Input: part model. Units: mm. Frame: model coordinates. Face numbers are marked on the shaded views. A direction names the side the tool comes from. Coordinates: 2 decimals unless noted, no trailing zeros. Write each loop counter-clockwise with the first axis right and the second up, starting at its lowest first coordinate (ties: lowest second). Pieces come first, ordered by that corner, then holes. Notation, with made-up numbers: (41.25, 74) - (100.25, 74) arc R11 cw to (100.25, 82) - close; hole circle Ø9 at (12.25, 77.25). An arc over 180 degrees is marked (long way). Use CSV: the item, a comma, the result in double quotes.
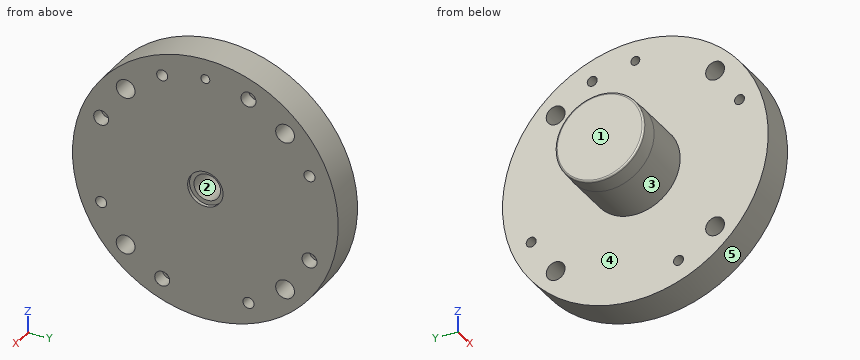
```python
from build123d import *

# Parameters (mm, degrees)
F2_R             = 6.7437
F3_DEPTH         = 25.4
F3_COPIES_COUNT  = 4
F8_COPIES_COUNT  = 4
F11_COPIES_COUNT = 4
F12_R            = 3.175
F13_DEPTH        = 25.4


# Not quite as in the source:
# - a pattern or mirror of a feature is missing from the dataset's text; its kind, count and spacing are read off the source's solid


with BuildPart() as f1:
    # F0 (on Front) → F1 (revolve)
    with BuildSketch(Plane.XZ):
        with BuildLine():
            Line((-46.99, 30.4610814834), (-46.99, 0))
            Line((-46.99, 0), (25.4, 0))
            Line((25.4, 0), (25.4, 95.25))
            Line((25.4, 95.25), (0, 95.25))
            Line((0, 95.25), (0, 32.131))
            Line((0, 32.131), (-34.29, 32.131))
            Line((-34.29, 32.131), (-45.7643223608, 31.7303078338))
            ThreePointArc((-45.7643223608, 31.7303078338), (-46.6335615464, 31.3432976139), (-46.99, 30.4610814834))
        make_face()
    revolve(axis=Axis((-33.2340214019, 0, 0), (-1, 0, 0)))

    # F2 (on Right) → F3 (cut, through all)
    with BuildSketch(Plane.YZ):
        with Locations((57.15, 57.15)):
            Circle(F2_R)
    f3 = extrude(amount=F3_DEPTH, mode=Mode.SUBTRACT)

    # F3_copies: F3 ×4 about axis
    f3_copies_axis = Axis((0, 0, 0), (1, 0, 0))
    for i in range(1, F3_COPIES_COUNT):
        add(f3.rotate(f3_copies_axis, i * 360 / F3_COPIES_COUNT), mode=Mode.SUBTRACT)

    # F4 (on Front) → F5 (revolve, cut)
    with BuildSketch(Plane.XZ):
        Polygon((-38.0918026038, 9.525), (-43.815, 0), (25.4, 0), (25.4, 12.7), (22.86, 12.7), (22.86, 9.525), align=None)
    revolve(axis=Axis((25.4, 0, 0), (1, 0, 0)), mode=Mode.SUBTRACT)

    # F7 (on line) → F8 (revolve, cut)
    with BuildSketch(Plane(origin=(0, 0, 0), x_dir=(-1, 0, 0), z_dir=(0, 0.9238795325, -0.3826834324))):
        Polygon((-25.4, 80.8228), (0, 80.8228), (0, 84.3915), (-15.494, 84.3915), (-15.494, 86.1822), (-25.4, 86.1822), align=None)
    f8 = revolve(axis=Axis((19.0941668783, 30.9295465174, 74.6705306803), (-1, 0, 0)), mode=Mode.SUBTRACT)

    # F8_copies: F8 ×4 about axis
    f8_copies_axis = Axis((0, 0, 0), (1, 0, 0))
    for i in range(1, F8_COPIES_COUNT):
        add(f8.rotate(f8_copies_axis, i * 360 / F8_COPIES_COUNT), mode=Mode.SUBTRACT)

    # F10 (on line) → F11 (revolve, cut)
    with BuildSketch(Plane(origin=(0, 0, 0), x_dir=(-1, 0, 0), z_dir=(0, 0.9238795325, 0.3826834324))):
        Polygon((-25.4, 84.79155), (-25.4, 80.8228), (-2.9182675346, 80.8228), (-4.826, 83.9978), (-7.9248, 83.9978), (-7.9248, 84.79155), align=None)
    f11 = revolve(axis=Axis((19.9955312124, -30.9295465174, 74.6705306803), (-1, 0, 0)), mode=Mode.SUBTRACT)

    # F11_copies: F11 ×4 about axis
    f11_copies_axis = Axis((0, 0, 0), (1, 0, 0))
    for i in range(1, F11_COPIES_COUNT):
        add(f11.rotate(f11_copies_axis, i * 360 / F11_COPIES_COUNT), mode=Mode.SUBTRACT)

    # F12 (on Right) → F13 (cut, through all)
    with BuildSketch(Plane.YZ):
        with Locations((0, 80.8228)):
            Circle(F12_R)
    extrude(amount=F13_DEPTH, mode=Mode.SUBTRACT)


solid = f1.part
```
(1) Reachability of the marked faces 4 and 5 from +Z, -Z, +X, -X, +Y, -Y: full face, straight path, thin tool, end or side. Return the list, or none.
Check values:
face 4,"-X"
face 5,"+X, -X"
(2) Cut plane A-A on z = 57.15. Return loops of the section in (x, y), and give its area (3 significant figures).
Check values:
outline,"(0, -76.2) - (25.4, -76.2) - (25.4, -63.89) - (0, -63.89) - close; (0, -50.41) - (25.4, -50.41) - (25.4, 50.41) - (0, 50.41) - close; (0, 63.89) - (25.4, 63.89) - (25.4, 76.2) - (0, 76.2) - close"
area,"3,190 mm^2"
(3) Cut plane C-C on x = 19. State how many separate pieces and enclosed holes the cut face has, and give its area (3 significant figures).
Check values:
separate pieces,"1"
enclosed holes,"14"
area,"27,100 mm^2"
(4) Ray query, probe 1 along Y at (x, z) = (9, 56.5); probe 2 along Z at (x, y) = (-17.5, 29.5); probe 3 along X at (y, z) = (49.5, -64). Return the intervals inside material, ascending. Write a range as from..to.
Check values:
probe 1,"-76.68..-63.86, -50.44..50.44, 63.86..76.68"
probe 2,"-12.73..12.73"
probe 3,"0..25.4"
(5) Pin query (flat end, axial travel): pin 1 Ø4 at (x, y) = (-38.5, 7) entering from +Z; pin 2 Ø2 at (x, y) = (-36, 14.5) entering from +Z; pin 3 Ø8 at (y, z) = (6, -3) entering from +X. Return the tip coordinate at first contact, or that it passes through.
Check values:
pin 1,"z = 31.6"
pin 2,"z = 29.09"
pin 3,"x = 22.86"
(6) Cut plane D-D on x = -14. Return loops of the section in (y, z) (3 decimals).
Check values:
outline,"circle Ø64.262 at (0, 0); hole circle Ø19.05 at (0, 0)"
(7) Cut plane B-B on y = -53.5. Return loops of the section in (x, z), and give its area (3 significant figures).
Check values:
outline,"(0, -78.81) - (25.4, -78.81) - (25.4, -62.82) - (0, -62.82) - close; (0, -51.48) - (25.4, -51.48) - (25.4, 51.48) - (0, 51.48) - close; (0, 62.82) - (25.4, 62.82) - (25.4, 78.81) - (0, 78.81) - close"
area,"3,430 mm^2"
(8) Draft query along Y for the marked faces 1, 2 and 3. Return one class per face: pulls with the +Y half, pulls with the -Y half, needs draft (parallel to the pull), parting line crosses it, or undercut.
Check values:
face 1,"needs draft"
face 2,"undercut"
face 3,"parting line crosses it"
